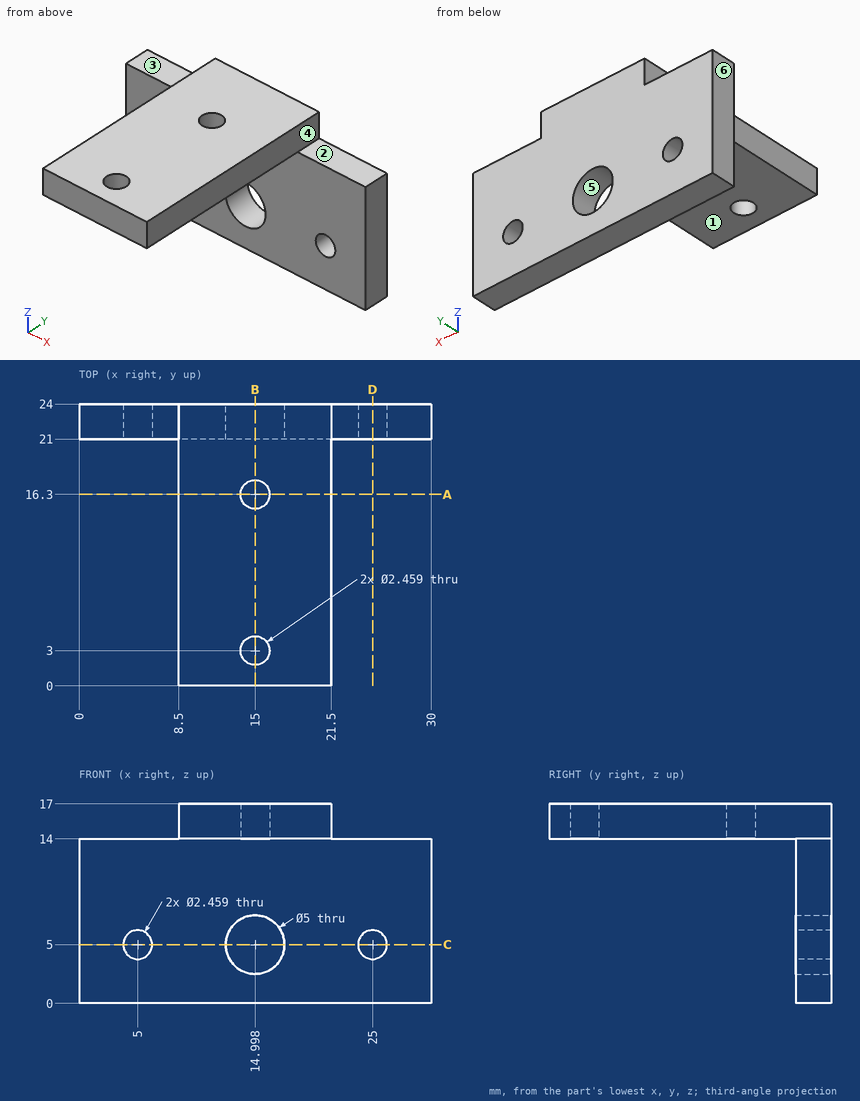
Design review of the part shown in the three views and the two pictorial views. Dimensions are in mm from the part's minimum x, y and z. A direction names the side the tool comes from. Round coordinates to 2 decimals unless told otherwise and drop trailing zeros. Order: outer loops, then holes, each group sorted by start corner. A loop starts at its lowest first (then second) coordinate and runs counter-clockwise, first axis right, second up.
(1) Mouldability with a two-part tool opening along X and no side actions: class the marked faces 4, 5 and 6 as released by +X, released by -X, zero draft, split by the parting line, or undercut.
Working result:
face 4: released by +X
face 5: undercut
face 6: released by -X
(2) For P1, Ø6, axis at y = 15.5, z = 12, coming from the -X side; P2, Ø4, axis at x = 5, z = 5, coming from the +Y side; P3, Ø4, axis at x = 19.5, y = 16.5, coming from the -Z side; P4, Ø2.5, axis at x = 24, y = 22.5, coming from the +Z side, all flat-tipped, find the tip position at first contact; note any pin that passes through.
Working result:
P1: stops at x = 8.5
P2: stops at y = 24
P3: stops at z = 14
P4: stops at z = 14
(3) Take a section at B-B, the plane x = 15. State the section outline as (y, z) points.
Working result:
outline: (0, 14) - (1.77, 14) - (1.77, 17) - (0, 17) - close; (4.23, 14) - (15.07, 14) - (15.07, 17) - (4.23, 17) - close; (17.53, 14) - (21, 14) - (21, 7.5) - (24, 7.5) - (24, 17) - (17.53, 17) - close; (21, 0) - (24, 0) - (24, 2.5) - (21, 2.5) - close
(4) Tool access review of the marked faces 1, 2 and 3: name each direction out of +Z, -Z, +X, -X, +Y, -Y from which nothing blocks a thin tool from reaching the whole face with its end or side.
Working result:
face 1: -Z, +X, -X, -Y
face 2: +Z, +X, +Y, -Y
face 3: +Z, -X, +Y, -Y
(5) Wall thickness on L1, parallel to X at y = 21.75, z = 5; L2, parallel to Y at x = 15, z = 15.55; L3, parallel to Z at x = 25, y = 21.65: over which ranges is each line inside the solid? List them lowest first.
Working result:
L1: x = 0 to 3.77, 6.23 to 12.5, 17.5 to 23.77, 26.23 to 30
L2: y = 0 to 1.77, 4.23 to 15.07, 17.53 to 24
L3: z = 0 to 3.77, 6.23 to 14
(6) Take a section at C-C, the plane z = 5. State the section outline as (x, y) points.
Working result:
outline: (0, 21) - (3.77, 21) - (3.77, 24) - (0, 24) - close; (6.23, 21) - (12.5, 21) - (12.5, 24) - (6.23, 24) - close; (17.5, 21) - (23.77, 21) - (23.77, 24) - (17.5, 24) - close; (26.23, 21) - (30, 21) - (30, 24) - (26.23, 24) - close
(7) Take a section at A-A, the plane y = 16.3. State the section outline as (x, z) points, plus the area to 3 significant figures.
Working result:
outline: (8.5, 14) - (13.77, 14) - (13.77, 17) - (8.5, 17) - close; (16.23, 14) - (21.5, 14) - (21.5, 17) - (16.23, 17) - close
area: 31.6 mm2
(8) Take a section at D-D, the plane x = 25. State the section outline as (y, z) points.
Working result:
outline: (21, 0) - (24, 0) - (24, 3.77) - (21, 3.77) - close; (21, 6.23) - (24, 6.23) - (24, 14) - (21, 14) - close
